Design review of the part built by this model. Coordinates are the model's own, in mm. A direction names the side the tool comes from. Round coordinates to 2 decimals unless told otherwise and drop trailing zeros. Loops run counter-clockwise (first coordinate to the right, second up) from the corner with the lowest first, then second, coordinate; pieces in that order, holes last. Notation, with made-up numbers: M 39,11.25 L 93,11.25 A20 cw 93,45.25 Z; hole C 72,54 d11. An arc over 180 degrees is marked long. Use a Markdown table: item, result.
from build123d import *

# Parameters (mm, degrees)
BOSS_EXTRUDE1_DEPTH = 4.5
BOSS_EXTRUDE2_DEPTH = 1


with BuildPart() as part:
    # Sketch1 → Boss-Extrude1 (new body)
    with BuildSketch(Plane.XY):
        Polygon((4.032829212, -1.498375708), (12.993598728, -1.498375708), (8.51321397, 6.26187833), align=None)
    extrude(amount=BOSS_EXTRUDE1_DEPTH)

    # Sketch2 → Boss-Extrude2 (add)
    with BuildSketch(Plane(origin=(0, 0, 0), x_dir=(-1, 0, 0), z_dir=(0, 0, -1))):
        Polygon((-14.817507964, 3.342520827), (-12.219431753, 1.842520827), (-14.725649535, -2.498375708), (-9.71321397, -2.498375708), (-9.71321397, -5.498375708), (-7.31321397, -5.498375708), (-7.31321397, -2.498375708), (-2.300778405, -2.498375708), (-4.806996187, 1.842520827), (-2.208919976, 3.342520827), (-3.408919976, 5.420981796), (-6.006996187, 3.920981796), (-8.51321397, 8.26187833), (-11.019431753, 3.920981796), (-13.617507964, 5.420981796), align=None)
    extrude(amount=BOSS_EXTRUDE2_DEPTH)


solid = part.part
1. Insertion check: pin 1 (1 mm diameter, centred on x = 4.5, z = 2, fed in from +Y); pin 2 (1.1 mm diameter, centred on y = -3.5, z = -0.5, fed in from -X); pin 3 (0.5 mm diameter, centred on y = -4.5, z = -0.5, fed in from +X). Each pin has a flat end and moves straight along its axis. Give the tip position at first contact, or say it passes through.
Check values:
| item | result |
|---|---|
| pin 1 | stops at y = 0.18 |
| pin 2 | stops at x = 7.31 |
| pin 3 | stops at x = 9.71 |
2. The part is to be moulded in two halves that separate along Y. For faces 1 (the face through (9.75, 6.12, -0.49)), 2 (the face through (4.8, -2.498, -0.5)), 3 (the face through (13.537, 2.603, -0.493)), say which applies: pulls with the +Y half, pulls with the -Y half, needs draft (parallel to the pull), parting line crosses it, or undercut.
Check values:
| item | result |
|---|---|
| face 1 | pulls with the +Y half |
| face 2 | pulls with the -Y half |
| face 3 | undercut |
3. Take a section at D-D on x = 8.75. Give the boundary of the cut face in (y, z), and give its area (3 significant figures).
Check values:
| item | result |
|---|---|
| outline | M -5.5,-1 L 7.85,-1 L 7.85,0 L 5.85,0 L 5.85,4.5 L -1.5,4.5 L -1.5,0 L -5.5,0 Z |
| area | 46.4 mm² |
4. Machinability: for faces 4 (the face through (3.53, 2.58, -0.49)), 5 (the face through (13.455, -0.298, -0.493)), 6 (the face through (6.304, 2.436, 2.218)), 7 (the face through (7.24, 6.06, -0.49)), which of the approach directions +Z, -Z, +X, -X, +Y, -Y give a long, thin tool a straight path to every point of the face, cutting with its end or side? Answer none if there is none.
Check values:
| item | result |
|---|---|
| face 4 | +Z, -Z, -X |
| face 5 | +Z, -Z, +X |
| face 6 | +Z, -X, +Y |
| face 7 | +Z, -Z, +Y |
5. Take a section at C-C on y = 2. Give the boundary of the cut face in (x, z), and give its area (3 significant figures).
Check values:
| item | result |
|---|---|
| outline | M 4.53,-1 L 12.49,-1 L 12.49,0 L 10.97,0 L 10.97,4.5 L 6.05,4.5 L 6.05,0 L 4.53,0 Z |
| area | 30.1 mm² |
6. Wall thickness on line 1 along Z through (x, y) = (8.5, -3.5); line 2 along Y through (x, z) = (9, 1.6); line 3 along Y through (x, z) = (6, 2.5): over which ranges is each line inside the solid? List them lowest first. Write a range as from..to.
Check values:
| item | result |
|---|---|
| line 1 | z = -1..0 |
| line 2 | y = -1.5..5.42 |
| line 3 | y = -1.5..1.91 |
7. Take a section at A-A on z = -0.6. Give the boundary of the cut face in (x, y), and give its area (3 significant figures).
Check values:
| item | result |
|---|---|
| outline | M 2.21,3.34 L 4.81,1.84 L 2.3,-2.5 L 7.31,-2.5 L 7.31,-5.5 L 9.71,-5.5 L 9.71,-2.5 L 14.73,-2.5 L 12.22,1.84 L 14.82,3.34 L 13.62,5.42 L 11.02,3.92 L 8.51,8.26 L 6.01,3.92 L 3.41,5.42 Z |
| area | 88.4 mm² |
8. Take a section at B-B on x = 4.25. Give the boundary of the cut face in (y, z), and give its area (3 significant figures).
Check values:
| item | result |
|---|---|
| outline | M -2.5,-1 L 0.88,-1 L 0.88,0 L -1.12,0 L -1.12,4.5 L -1.5,4.5 L -1.5,0 L -2.5,0 Z; M 2.16,-1 L 4.94,-1 L 4.94,0 L 2.16,0 Z |
| area | 7.84 mm² |
